The listing builds one solid part. Answer for the finished solid, in the listing's coordinates (mm). Give positions to 0.01 mm unless a question says otherwise; leave off trailing zeros. Loops run counter-clockwise (first coordinate to the right, second up) from the corner with the lowest first, then second, coordinate; pieces in that order, holes last. Notation, with made-up numbers: M -17,44 L 20,44 A8 ccw 20,58 Z; hole C -13.5,25 d10. An arc over 180 degrees is marked long. Return JSON: item names as keys, results as strings.
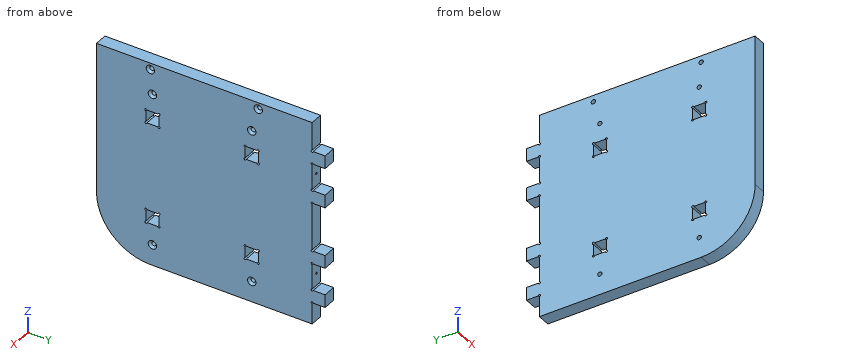
from build123d import *

# Parameters (mm, degrees)
SKETCH1_R                 = 2
SKETCH1_W                 = 12.1
SKETCH1_H                 = 12.1
BOSS_EXTRUDE1_DEPTH       = 12
CUT_EXTRUDE2_START        = 103.950538
SKETCH4_R                 = 0.9921875
CUT_EXTRUDE2_DEPTH        = 15
SKETCH5_R                 = 1
CUT_EXTRUDE3_DEPTH        = 15
ADVANCEDHOLE2_OUTLINE_R   = 1.89865
ADVANCEDHOLE2_DEPTH       = 2.301024407
ADVANCEDHOLE2_DRAFT       = -41
ADVANCEDHOLE2_2_OUTLINE_R = 1.89865
ADVANCEDHOLE2_2_DEPTH     = 2.301024407
ADVANCEDHOLE2_2_DRAFT     = -41
SKETCH8_R                 = 2
CUT_EXTRUDE4_DEPTH        = 154.260488233


# Read off the part's stored shape, not the designer's step: AdvancedHole1, AdvancedHole2
with BuildPart() as part:
    # Sketch1 → Boss-Extrude1 (new body)
    with BuildSketch(Plane(origin=(0, 0, 0), x_dir=(0, 0, -1), z_dir=(1, 0, 0))):
        with BuildLine():
            Line((-72.5, 115.950537961), (-72.5, 103.950537961))
            Line((-72.5, 103.950537961), (-99.5, 103.950537961))
            Line((-99.5, 103.950537961), (-99.5, -96.049462039))
            Line((-99.5, -96.049462039), (40.5, -96.049462039))
            ThreePointArc((40.5, -96.049462039), (75.855339059, -81.404801099), (90.5, -46.049462039))
            Line((90.5, -46.049462039), (90.5, 103.950537961))
            Line((90.5, 103.950537961), (70.5, 103.950537961))
            Line((70.5, 103.950537961), (70.5, 115.950537961))
            Line((70.5, 115.950537961), (58.5, 115.950537961))
            Line((58.5, 115.950537961), (58.5, 103.950537961))
            Line((58.5, 103.950537961), (33.5, 103.950537961))
            Line((33.5, 103.950537961), (33.5, 115.950537961))
            Line((33.5, 115.950537961), (21.5, 115.950537961))
            Line((21.5, 115.950537961), (21.5, 103.950537961))
            Line((21.5, 103.950537961), (-23.5, 103.950537961))
            Line((-23.5, 103.950537961), (-23.5, 115.950537961))
            Line((-23.5, 115.950537961), (-35.5, 115.950537961))
            Line((-35.5, 115.950537961), (-35.5, 103.950537961))
            Line((-35.5, 103.950537961), (-60.5, 103.950537961))
            Line((-60.5, 103.950537961), (-60.5, 115.950537961))
            Line((-60.5, 115.950537961), (-72.5, 115.950537961))
        make_face()
        with Locations((71.25, 47.900537961)):
            Circle(SKETCH1_R, mode=Mode.SUBTRACT)
        with Locations((71.25, -44.199462039)):
            Circle(SKETCH1_R, mode=Mode.SUBTRACT)
        with Locations((-70.75, 47.900537961)):
            Circle(SKETCH1_R, mode=Mode.SUBTRACT)
        with Locations((-70.75, -44.199462039)):
            Circle(SKETCH1_R, mode=Mode.SUBTRACT)
        with Locations((46, 47.900537961)):
            Rectangle(SKETCH1_W, SKETCH1_H, mode=Mode.SUBTRACT)
        with Locations((46, -44.199462039)):
            Rectangle(SKETCH1_W, SKETCH1_H, mode=Mode.SUBTRACT)
        with Locations((-48, 47.900537961)):
            Rectangle(SKETCH1_W, SKETCH1_H, mode=Mode.SUBTRACT)
        with Locations((-48, -44.199462039)):
            Rectangle(SKETCH1_W, SKETCH1_H, mode=Mode.SUBTRACT)
    extrude(amount=BOSS_EXTRUDE1_DEPTH)

    # Sketch4 → Cut-Extrude2 (cut)
    with BuildSketch(Plane(origin=(0, 0, 0), x_dir=(1, 0, 0), z_dir=(0, 1, 0)).offset(CUT_EXTRUDE2_START)):
        with Locations(Location((6, 46, 0), (0, 0, 90))):
            Circle(SKETCH4_R)
        with Locations(Location((6, -48, 0), (0, 0, 90))):
            Circle(SKETCH4_R)
    extrude(amount=-CUT_EXTRUDE2_DEPTH, mode=Mode.SUBTRACT)

    # Sketch5 → Cut-Extrude3 (cut)
    with BuildSketch(Plane(origin=(0, 0, 0), x_dir=(0, 0, -1), z_dir=(1, 0, 0))):
        with Locations((-54.05, 53.950537961)):
            Circle(SKETCH5_R)
        with Locations((-41.95, 53.950537961)):
            Circle(SKETCH5_R)
        with Locations((-41.95, 41.850537961)):
            Circle(SKETCH5_R)
        with Locations((-54.05, 41.850537961)):
            Circle(SKETCH5_R)
        with Locations((39.95, 53.950537961)):
            Circle(SKETCH5_R)
        with Locations((52.05, 53.950537961)):
            Circle(SKETCH5_R)
        with Locations((52.05, 41.850537961)):
            Circle(SKETCH5_R)
        with Locations((39.95, 41.850537961)):
            Circle(SKETCH5_R)
        with Locations((-41.95, -38.149462039)):
            Circle(SKETCH5_R)
        with Locations((-54.05, -38.149462039)):
            Circle(SKETCH5_R)
        with Locations((-41.95, -50.249462039)):
            Circle(SKETCH5_R)
        with Locations((-54.05, -50.249462039)):
            Circle(SKETCH5_R)
        with Locations((39.95, -38.149462039)):
            Circle(SKETCH5_R)
        with Locations((52.05, -38.149462039)):
            Circle(SKETCH5_R)
        with Locations((52.05, -50.249462039)):
            Circle(SKETCH5_R)
        with Locations((39.95, -50.249462039)):
            Circle(SKETCH5_R)
        with Locations((21.5, 103.950537961)):
            Circle(SKETCH5_R)
        with Locations((33.5, 103.950537961)):
            Circle(SKETCH5_R)
        with Locations((58.5, 103.950537961)):
            Circle(SKETCH5_R)
        with Locations((70.5, 103.950537961)):
            Circle(SKETCH5_R)
        with Locations((-23.5, 103.950537961)):
            Circle(SKETCH5_R)
        with Locations((-35.5, 103.950537961)):
            Circle(SKETCH5_R)
        with Locations((-60.5, 103.950537961)):
            Circle(SKETCH5_R)
        with Locations((-72.5, 103.950537961)):
            Circle(SKETCH5_R)
    extrude(amount=CUT_EXTRUDE3_DEPTH, mode=Mode.SUBTRACT)

    # AdvancedHole1 outline → AdvancedHole1 (revolve, cut)
    with BuildSketch(Plane(origin=(0, -44.199462039, 70.75), x_dir=(0, 1, 0), z_dir=(0, 0, -1))):
        Polygon((2, 12), (2, 9.815565432), (3.8989, 12), align=None)
    revolve(axis=Axis((0, -44.199462039, 70.75), (1, 0, 0)), mode=Mode.SUBTRACT)

    # AdvancedHole1 2 outline → AdvancedHole1 2 (revolve, cut)
    with BuildSketch(Plane(origin=(0, 47.900537961, 70.75), x_dir=(0, 1, 0), z_dir=(0, 0, -1))):
        Polygon((2, 12), (2, 9.815565432), (3.8989, 12), align=None)
    revolve(axis=Axis((0, 47.900537961, 70.75), (1, 0, 0)), mode=Mode.SUBTRACT)

    # AdvancedHole1 3 outline → AdvancedHole1 3 (revolve, cut)
    with BuildSketch(Plane(origin=(0, -44.199462039, -71.25), x_dir=(0, 1, 0), z_dir=(0, 0, -1))):
        Polygon((2, 12), (2, 9.815565432), (3.8989, 12), align=None)
    revolve(axis=Axis((0, -44.199462039, -71.25), (1, 0, 0)), mode=Mode.SUBTRACT)

    # AdvancedHole1 4 outline → AdvancedHole1 4 (revolve, cut)
    with BuildSketch(Plane(origin=(0, 47.900537961, -71.25), x_dir=(0, 1, 0), z_dir=(0, 0, -1))):
        Polygon((2, 12), (2, 9.815565432), (3.8989, 12), align=None)
    revolve(axis=Axis((0, 47.900537961, -71.25), (1, 0, 0)), mode=Mode.SUBTRACT)


with BuildPart() as advancedhole2_tool:
    # AdvancedHole2 outline → AdvancedHole2 (with draft: the straight prism first)
    with BuildSketch(Plane.YZ.offset(9.698975593)):
        with Locations((-46.049462039, 93.5)):
            Circle(ADVANCEDHOLE2_OUTLINE_R)
    extrude(amount=ADVANCEDHOLE2_DEPTH)
    # AdvancedHole2: the draft: its side faces are tilted about the plane it starts from
    advancedhole2_sides = [advancedhole2_tool.faces().sort_by_distance(p)[0] for p in [
        (10.849487797, -47.948112039, 93.5),
    ]]
    draft(advancedhole2_sides, Plane.YZ.offset(9.698975593), ADVANCEDHOLE2_DRAFT)


with BuildPart() as part_1:
    add(part.part)

    # AdvancedHole2: cut by advancedhole2_tool
    add(advancedhole2_tool.part, mode=Mode.SUBTRACT)


with BuildPart() as advancedhole2_2_tool:
    # AdvancedHole2 2 outline → AdvancedHole2 2 (with draft: the straight prism first)
    with BuildSketch(Plane.YZ.offset(9.698975593)):
        with Locations((53.950537961, 93.5)):
            Circle(ADVANCEDHOLE2_2_OUTLINE_R)
    extrude(amount=ADVANCEDHOLE2_2_DEPTH)
    # AdvancedHole2 2: the draft: its side faces are tilted about the plane it starts from
    advancedhole2_2_sides = [advancedhole2_2_tool.faces().sort_by_distance(p)[0] for p in [
        (10.849487797, 52.051887961, 93.5),
    ]]
    draft(advancedhole2_2_sides, Plane.YZ.offset(9.698975593), ADVANCEDHOLE2_2_DRAFT)


with BuildPart() as part_2:
    add(part_1.part)

    # AdvancedHole2 2: cut by advancedhole2_2_tool
    add(advancedhole2_2_tool.part, mode=Mode.SUBTRACT)

    # Sketch8 → Cut-Extrude4 (cut, through all)
    with BuildSketch(Plane(origin=(12, 0, 0), x_dir=(0, 0, -1), z_dir=(1, 0, 0))):
        with Locations((-93.5, 53.950537961)):
            Circle(SKETCH8_R)
        with Locations((-93.5, -46.049462039)):
            Circle(SKETCH8_R)
    extrude(amount=-CUT_EXTRUDE4_DEPTH, mode=Mode.SUBTRACT)


solid = part_2.part
(1) The part is cut by section B-B (x = 2). Give the number of separate pieces and of enclosed holes in the cut face, and give its area (3 significant figures).
Values follow:
{"separate pieces": "1", "enclosed holes": "10", "area": "37,300 mm²"}
(2) Straight lines are drawn through the part: line 1 along Z through (x, y) = (6, 93.75); line 2 along Y through (x, z) = (6.75, 42); line 3 along Y through (x, z) = (4.75, 70.75). For each, find the intervals that lie inside material, in ascending order.
Values follow:
{"line 1": "-90.5 to -46.99, -45.01 to 47.01, 48.99 to 99.5", "line 2": "-96.05 to -51.25, -37.15 to 40.85, 54.95 to 103.95", "line 3": "-96.05 to -46.2, -42.2 to 45.9, 49.9 to 115.95"}
(3) Given pin 1 (3.5 mm diameter, centred on x = 4.5, z = 45, fed in from +Y); pin 2 (6 mm diameter, centred on x = 8, z = -64.5, fed in from -Y); pin 3 (5.5 mm diameter, centred on x = 9, y = 111, fed in from -Z), each flat-ended and moving along its own axis, determine where each tip first touches the part or whether it passes through.
Values follow:
{"pin 1": "y = 103.95", "pin 2": "y = -91.43", "pin 3": "z = -70.5"}
(4) The part is cut by section A-A (z = 8). Determine the outline of the cut face in (x, y), and give its area (3 significant figures).
Values follow:
{"outline": "M 0,-96.05 L 12,-96.05 L 12,103.95 L 0,103.95 Z", "area": "2,400 mm²"}
